Part print with two shaded views. Sizes in mm from the minimum x, y, z corner. A direction names the side the tool comes from. Round coordinates to 2 decimals unless told otherwise and drop trailing zeros. Loops run counter-clockwise (first coordinate to the right, second up) from the corner with the lowest first, then second, coordinate; pieces in that order, holes last. Notation, with made-up numbers: (16, 29) - (68, 29) arc R24 cw to (68, 65) - close; hole circle Ø1 at (-12, 50). An arc over 180 degrees is marked (long way). Use a Markdown table: item, result.
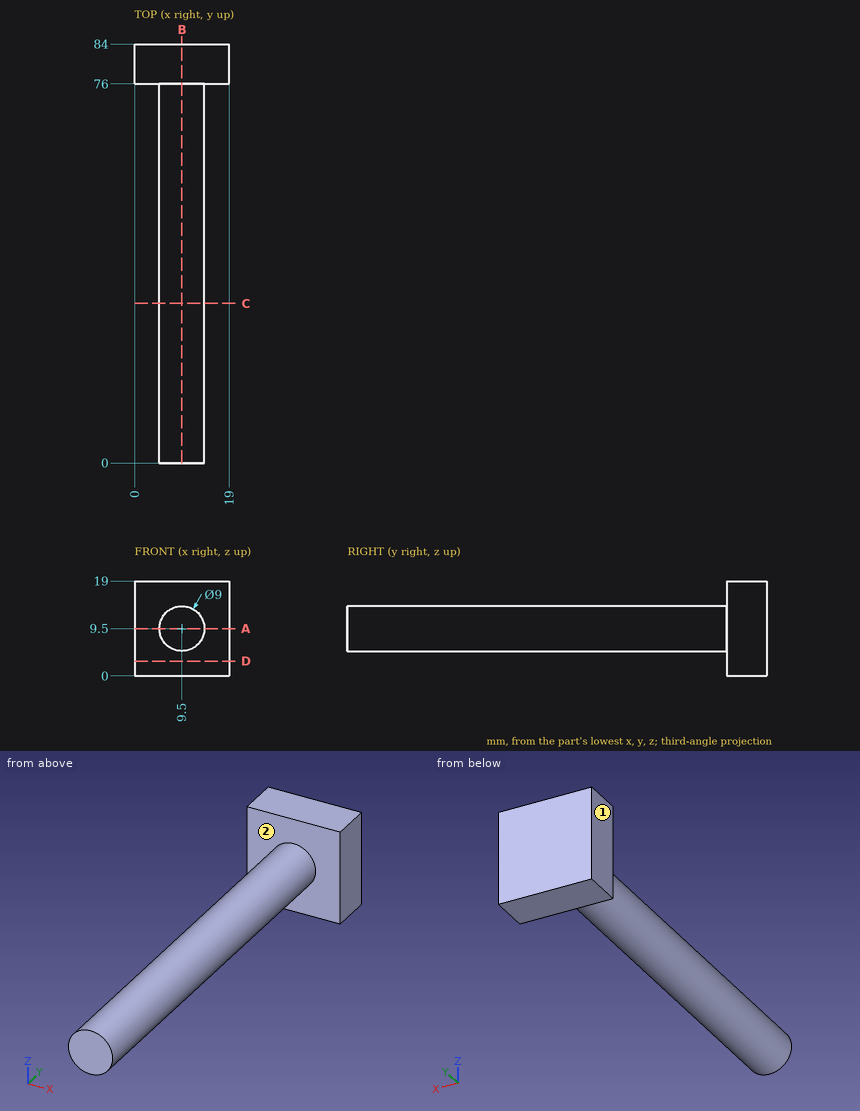
Q1. Cut at A-A, the plane z = 9.5. List the corners of the cut face in (x, y), plus the area to 3 significant figures.
Results found:
| item | result |
|---|---|
| outline | (0, 76) - (5, 76) - (5, 0) - (14, 0) - (14, 76) - (19, 76) - (19, 84) - (0, 84) - close |
| area | 836 mm2 |
Q2. Cut at C-C, the plane y = 32. List the corners of the cut face in (x, z).
Results found:
| item | result |
|---|---|
| outline | circle Ø9 at (9.5, 9.5) |
Q3. Probe line 1 (Y direction, x = 16.75, z = 11); line 2 (Z direction, x = 13, y = 59); line 3 (X direction, y = 25.5, z = 10.5). List the from-to ranges inside material, lowest first.
Results found:
| item | result |
|---|---|
| line 1 | y = 76 to 84 |
| line 2 | z = 6.67 to 12.33 |
| line 3 | x = 5.11 to 13.89 |
Q4. Cut at B-B, the plane x = 9.5. List the corners of the cut face in (y, z).
Results found:
| item | result |
|---|---|
| outline | (0, 5) - (76, 5) - (76, 0) - (84, 0) - (84, 19) - (76, 19) - (76, 14) - (0, 14) - close |
Q5. Drop flat-ended pins along their axis: pin 1 (5 mm diameter, centred on x = 5, y = 16, fed in from +Z); pin 2 (5 mm diameter, centred on y = 34.5, z = 16, fed in from -X); pin 3 (1 mm diameter, centred on x = 13.5, z = 16, fed in from -Y). Give the stop position or say it passes through.
Results found:
| item | result |
|---|---|
| pin 1 | stops at z = 13.53 |
| pin 2 | stops at x = 7.44 |
| pin 3 | stops at y = 76 |
Q6. Cut at D-D, the plane z = 3. List the corners of the cut face in (x, y).
Results found:
| item | result |
|---|---|
| outline | (0, 76) - (19, 76) - (19, 84) - (0, 84) - close |
Q7. Which spindle directions (+Z, -Z, +X, -X, +Y, -Y) get a long thin tool onto all of the face, cutting with end or side? Do the marked faces 1 and 2. Say none if no direction does.
Results found:
| item | result |
|---|---|
| face 1 | +Z, -Z, -X, +Y, -Y |
| face 2 | -Y |
